Could you check a few things on this model? Use its own coordinates, in mm. Round coordinates to 2 decimals unless told otherwise and drop trailing zeros. Write each loop counter-clockwise with the first axis right and the second up, starting at its lowest first coordinate (ties: lowest second). Pieces come first, ordered by that corner, then holes. Notation, with made-up numbers: (-34, -28) -> (-27, -28) arc R13 ccw to (-27, -14) -> close; hole circle Ø6 at (41, 70). An arc over 180 degrees is marked (long way). Return JSON: item names as keys, results as strings.
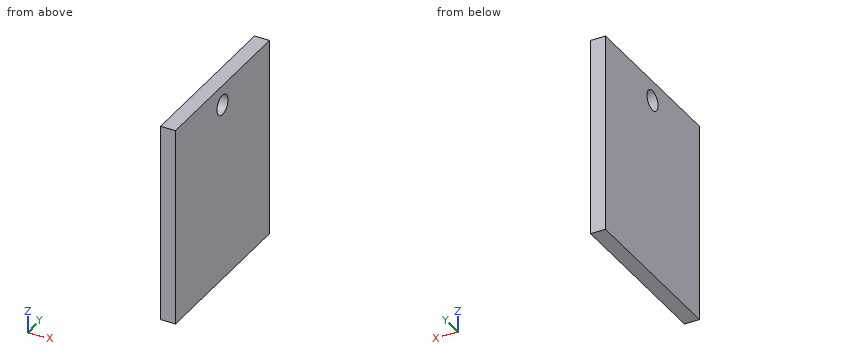
Autodesk Inventor part; units mm, degrees
ref_plane "YZ Plane" through (0, 0, 0) normal (1, 0, 0) x (0, 1, 0)
ref_plane "XZ Plane" through (0, 0, 0) normal (0, 1, 0) x (-1, 0, 0)
ref_plane "XY Plane" through (0, 0, 0) normal (0, 0, 1) x (1, 0, 0)
ref_plane "Work Plane1" through (0, 0, 0) normal (0, 0, 1) x (1, 0, 0)
sketch "Sketch1" plane through (0, 0, 0) normal (0, 0, 1) x (1, 0, 0)
  circle A0 centre (0, 0) radius 152.4
  line L0 (107.95, -107.5758) -> (107.95, 107.5758)
  line L1 (88.9, 107.5758) -> (88.9, -107.5758)
  line L2 (88.9, -107.5758) -> (107.95, -107.5758)
  line L3 (88.9, 107.5758) -> (107.95, 107.5758)
  dimension "d0" = 19.05
  dimension "d1" = 88.9
extrude "Extrusion1" add sketch "Sketch1" along normal blind 254 contours L0 L2 L1 L3
sketch "Sketch2" plane through (107.95, -107.5758, 0) normal (1, 0, 0) x (0, 0, -1)
  line L0 (-254, 0) -> (-254, 215.1516) construction
  line L1 (-254, 107.5758) -> (0, 107.5758) construction
  circle A0 centre (-228.6, 107.5758) radius 12.7
  dimension "d4" = 25.4
  dimension "d5" = 25.4
extrude "Extrusion2" cut sketch "Sketch2" against normal through all
properties part number "sideSupportFor12inchBase"
1) I want a section at A-A, the plane y = 0. Please give me the cut outline in (x, z), and give its area (3 significant figures).
Return value:
{"outline": "(88.9, 0) -> (107.95, 0) -> (107.95, 215.9) -> (88.9, 215.9) -> close; (88.9, 241.3) -> (107.95, 241.3) -> (107.95, 254) -> (88.9, 254) -> close", "area": "4,350 mm²"}
2) If I drill on probe 1 along Y at (x, z) = (103.25, 228.6); probe 2 along Y at (x, z) = (99.5, 225), over which ranges is the centre line in solid material (lowest first)? Write a range as [from, to].
Return value:
{"probe 1": "[-107.58, -12.7], [12.7, 107.58]", "probe 2": "[-107.58, -12.18], [12.18, 107.58]"}
3) I want a section at B-B, the plane z = 228.6. Please give me the cut outline in (x, y).
Return value:
{"outline": "(88.9, -107.58) -> (107.95, -107.58) -> (107.95, -12.7) -> (88.9, -12.7) -> close; (88.9, 12.7) -> (107.95, 12.7) -> (107.95, 107.58) -> (88.9, 107.58) -> close"}
